from build123d import *

# Parameters (mm, degrees)
BOSS_EXTRUDE1_DEPTH                             = 4.7625
SKETCH9_W                                       = 6.5
SKETCH9_H                                       = 3.175
CUT_EXTRUDE2_DEPTH                              = 50.705949405
CSK_FOR_M2_FLAT_HEAD_MACHINE_SCREW1_D           = 2.4
CSK_FOR_M2_FLAT_HEAD_MACHINE_SCREW1_DEPTH       = 3.175
CSK_FOR_M2_FLAT_HEAD_MACHINE_SCREW1_CSINK_D     = 4.4
CSK_FOR_M2_FLAT_HEAD_MACHINE_SCREW1_CSINK_ANGLE = 90
M2X0_4_TAPPED_HOLE1_D                           = 1.6


with BuildPart() as part:
    # Sketch1 → Boss-Extrude1 (new, symmetric)
    with BuildSketch(Plane(origin=(0, 0, 0), x_dir=(1, 0, 0), z_dir=(0, 1, 0))):
        with BuildLine():
            Line((-24, 0), (24, 0))
            Line((24, 0), (24, -12))
            ThreePointArc((24, -12), (0, -9.077288796), (-24, -12))
            Line((-24, -12), (-24, 0))
        make_face()
    extrude(amount=BOSS_EXTRUDE1_DEPTH, both=True)

    # Sketch9 → Cut-Extrude2 (cut, through all)
    with BuildSketch(Plane.ZY.offset(24)):
        with Locations((3.25, 0)):
            Rectangle(SKETCH9_W, SKETCH9_H)
    extrude(amount=-CUT_EXTRUDE2_DEPTH, mode=Mode.SUBTRACT)

    # CSK for M2 Flat Head Machine Screw1
    with Locations(Plane(origin=(0, 4.7625, 0), x_dir=(1, 0, 0), z_dir=(0, 1, 0))):
        with Locations((-12.5, -4), (12.5, -4)):
            CounterSinkHole(CSK_FOR_M2_FLAT_HEAD_MACHINE_SCREW1_D / 2, CSK_FOR_M2_FLAT_HEAD_MACHINE_SCREW1_CSINK_D / 2, depth=CSK_FOR_M2_FLAT_HEAD_MACHINE_SCREW1_DEPTH, counter_sink_angle=CSK_FOR_M2_FLAT_HEAD_MACHINE_SCREW1_CSINK_ANGLE)

    # M2x0.4 Tapped Hole1 (through all)
    with Locations(Plane(origin=(0, -1.5875, 0), x_dir=(1, 0, 0), z_dir=(0, 1, 0))):
        with Locations((-12.5, -4), (12.5, -4)):
            Hole(M2X0_4_TAPPED_HOLE1_D / 2)


solid = part.part
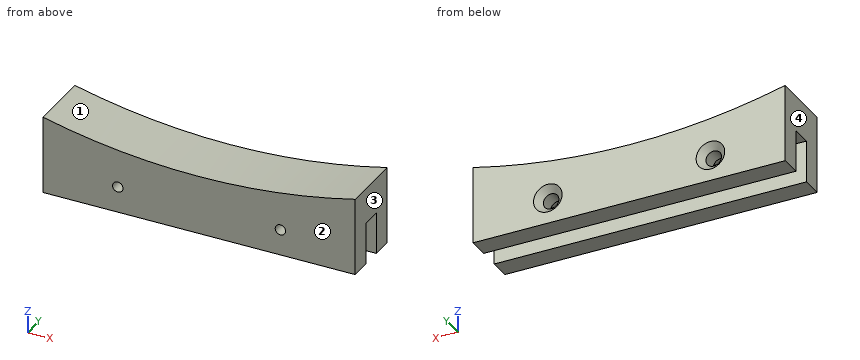
Model file for the job. Use its own axes, mm. Face numbers are marked on the shaded views. Give positions to 0.01 mm unless a question says otherwise; leave off trailing zeros. Order: outer loops, then holes, each group sorted by start corner. A loop starts at its lowest first (then second) coordinate and runs counter-clockwise, first axis right, second up. Notation, with made-up numbers: (78, -30.5) - (122, -30.5) arc R30 ccw to (122, -0.5) - close; hole circle Ø7 at (14, -29.75). An arc over 180 degrees is marked (long way). Return JSON: item names as keys, results as strings.
1) Flat gauge pins, fed straight in: P1, Ø1.5, axis at x = -0.5, y = -3, coming from the +Z side; P2, Ø1, axis at x = 12.5, z = 4, coming from the +Y side (3 decimals); P3, Ø1, axis at x = -8.5, y = -1, coming from the -Z side; P4, Ø3, axis at x = -12.5, z = 4, coming from the +Y side. Where does each tip first touch, or does it go through?
Geometry says:
{"P1": "z = 9.09", "P2": "through", "P3": "z = 6.5", "P4": "y = 4.06"}
2) Probe line 1 (X direction, y = 2.55, z = 4); line 2 (X direction, y = -2.95, z = 4); line 3 (Y direction, x = -12, z = 0.75). List the from-to ranges inside material, lowest first. Write a range as from..to.
Geometry says:
{"line 1": "-24..-13.7, -11.3..11.3, 13.7..24", "line 2": "-24..-13.3, -11.7..11.7, 13.3..24", "line 3": "-4.76..-1.59, 1.59..4.76"}
3) Cut at C-C, the plane x = -12.5. Give the cut face in (y, z), plus the area to 3 significant figures.
Geometry says:
{"outline": "(-4.76, 0) - (-1.59, 0) - (-1.59, 3.2) - (-4.76, 3.2) - close; (-4.76, 4.8) - (-1.59, 4.8) - (-1.59, 6.5) - (1.59, 6.5) - (1.59, 5.2) - (3.76, 5.2) - (4.76, 6.2) - (4.76, 9.86) - (-4.76, 9.86) - close; (1.59, 0) - (4.76, 0) - (4.76, 1.8) - (3.76, 2.8) - (1.59, 2.8) - close", "area": "59.6 mm²"}
4) Cut at D-D, the plane x = 4. Give the cut face in (y, z).
Geometry says:
{"outline": "(-4.76, 0) - (-1.59, 0) - (-1.59, 6.5) - (1.59, 6.5) - (1.59, 0) - (4.76, 0) - (4.76, 9.16) - (-4.76, 9.16) - close"}
5) Cut at B-B, the plane z = 11. Give the cut face in (x, y).
Geometry says:
{"outline": "(-24, -4.76) - (-19.52, -4.76) - (-19.52, 4.76) - (-24, 4.76) - close; (19.52, -4.76) - (24, -4.76) - (24, 4.76) - (19.52, 4.76) - close"}
6) Cut at A-A, the plane z = 4. Give the cut face in (x, y), plus the area to 3 significant figures.
Geometry says:
{"outline": "(-24, -4.76) - (-13.3, -4.76) - (-13.3, -1.59) - (-24, -1.59) - close; (-24, 1.59) - (-13.7, 1.59) - (-13.7, 3.76) - (-14.7, 4.76) - (-24, 4.76) - close; (-11.7, -4.76) - (11.7, -4.76) - (11.7, -1.59) - (-11.7, -1.59) - close; (-11.3, 1.59) - (11.3, 1.59) - (11.3, 3.76) - (10.3, 4.76) - (-10.3, 4.76) - (-11.3, 3.76) - close; (13.3, -4.76) - (24, -4.76) - (24, -1.59) - (13.3, -1.59) - close; (13.7, 1.59) - (24, 1.59) - (24, 4.76) - (14.7, 4.76) - (13.7, 3.76) - close", "area": "277 mm²"}
7) Pull direction X, two halves, no side cores. Call the marked faces 1, 2, 3 and 4: pulls with the +X half, pulls with the -X half, needs draft (parallel to the pull), parting line crosses it, or undercut.
Geometry says:
{"face 1": "undercut", "face 2": "needs draft", "face 3": "pulls with the +X half", "face 4": "pulls with the -X half"}
